For this review, take the finished solid that the model builds, in its own axes (mm). Round coordinates to 2 decimals unless told otherwise and drop trailing zeros. Loops run counter-clockwise (first coordinate to the right, second up) from the corner with the lowest first, then second, coordinate; pieces in that order, holes last.
1) Wall thickness on L1, parallel to X at y = 0.55, z = 19.05 (3 decimals); L2, parallel to Z at x = -28, y = 0.5; L3, parallel to Z at x = 45, y = 0.5: over which ranges is each line inside the solid? List them lowest first.
2) Take a section at A-A (x = -24.5). State the section outline as (y, z) points.
3) Insertion check: pin 1 (8 mm diameter, centred on x = -82.55, z = 39.37, fed in from +Y); pin 2 (3 mm diameter, centred on x = -64.21, z = -39.37, fed in from -Y). Each pin has a flat end and moves straight along its axis. Give the tip position at first contact, or say it passes through.
4) Take a section at B-B (z = 5.5). State the section outline as (x, y) points, then the cut area to 3 significant figures.
5) Take a section at C-C (z = 19.05). Give the number of separate pieces and of enclosed holes in the cut face, then the cut area to 3 significant figures.
```python
from build123d import *

# Parameters (mm, degrees)
SKETCH1_W           = 190.5
SKETCH1_H           = 114.3
BOSS_EXTRUDE1_DEPTH = 1.5875
SKETCH6_W           = 139.7
SKETCH6_H           = 63.5
CUT_EXTRUDE1_DEPTH  = 3.175
FILLET1_R           = 2.54
SKETCH7_R           = 3.175
CUT_EXTRUDE2_DEPTH  = 3.175
SKETCH8_R           = 2.54
CUT_EXTRUDE3_DEPTH  = 2.54
SKETCH9_R           = 2.54
CUT_EXTRUDE4_DEPTH  = 2.54
SKETCH10_W          = 68.58
SKETCH10_H          = 12.7
CUT_EXTRUDE5_DEPTH  = 112.090976934
FILLET2_R           = 2.54


with BuildPart() as part:
    # Sketch1 → Boss-Extrude1 (new body)
    with BuildSketch(Plane(origin=(0, 0, 0), x_dir=(1, 0, 0), z_dir=(0, 1, 0))):
        Rectangle(SKETCH1_W, SKETCH1_H)
    extrude(amount=BOSS_EXTRUDE1_DEPTH)

    # Sketch6 → Cut-Extrude1 (cut)
    with BuildSketch(Plane(origin=(0, 1.5875, 0), x_dir=(1, 0, 0), z_dir=(0, 1, 0))):
        Rectangle(SKETCH6_W, SKETCH6_H)
    extrude(amount=-CUT_EXTRUDE1_DEPTH, mode=Mode.SUBTRACT)

    # Fillet1
    fillet1_edges = [part.edges().sort_by_distance(p)[0] for p in [
        (-69.85, 0.79375, 31.75),
        (-69.85, 0.79375, -31.75),
        (69.85, 0.79375, -31.75),
        (69.85, 0.79375, 31.75),
        (95.25, 0.79375, -57.15),
        (95.25, 0.79375, 57.15),
        (-95.25, 0.79375, 57.15),
        (-95.25, 0.79375, -57.15),
    ]]
    fillet(fillet1_edges, radius=FILLET1_R)

    # Sketch7 → Cut-Extrude2 (cut)
    with BuildSketch(Plane(origin=(0, 1.5875, 0), x_dir=(1, 0, 0), z_dir=(0, 1, 0))):
        with Locations(Location((-82.55, 19.05, 0), (0, 0, 270))):
            Circle(SKETCH7_R)
        with Locations(Location((-82.55, -19.05, 0), (0, 0, 270))):
            Circle(SKETCH7_R)
        with Locations(Location((82.55, -19.05, 0), (0, 0, 270))):
            Circle(SKETCH7_R)
        with Locations(Location((82.55, 19.05, 0), (0, 0, 270))):
            Circle(SKETCH7_R)
    extrude(amount=-CUT_EXTRUDE2_DEPTH, mode=Mode.SUBTRACT)

    # Sketch8 → Cut-Extrude3 (cut)
    with BuildSketch(Plane(origin=(0, 1.5875, 0), x_dir=(1, 0, 0), z_dir=(0, 1, 0))):
        with Locations(Location((82.55, 39.37, 0), (0, 0, 270))):
            Circle(SKETCH8_R)
        with Locations(Location((64.205555556, 39.37, 0), (0, 0, 270))):
            Circle(SKETCH8_R)
        with Locations(Location((45.861111111, 39.37, 0), (0, 0, 270))):
            Circle(SKETCH8_R)
        with Locations(Location((27.516666667, 39.37, 0), (0, 0, 270))):
            Circle(SKETCH8_R)
        with Locations(Location((9.172222222, 39.37, 0), (0, 0, 270))):
            Circle(SKETCH8_R)
        with Locations(Location((-9.172222222, 39.37, 0), (0, 0, 270))):
            Circle(SKETCH8_R)
        with Locations(Location((-27.516666667, 39.37, 0), (0, 0, 270))):
            Circle(SKETCH8_R)
        with Locations(Location((-45.861111111, 39.37, 0), (0, 0, 270))):
            Circle(SKETCH8_R)
        with Locations(Location((-64.205555556, 39.37, 0), (0, 0, 270))):
            Circle(SKETCH8_R)
        with Locations(Location((-82.55, 39.37, 0), (0, 0, 270))):
            Circle(SKETCH8_R)
    extrude(amount=-CUT_EXTRUDE3_DEPTH, mode=Mode.SUBTRACT)

    # Sketch9 → Cut-Extrude4 (cut)
    with BuildSketch(Plane(origin=(0, 1.5875, 0), x_dir=(1, 0, 0), z_dir=(0, 1, 0))):
        with Locations(Location((82.55, -39.37, 0), (0, 0, 270))):
            Circle(SKETCH9_R)
        with Locations(Location((64.205555556, -39.37, 0), (0, 0, 270))):
            Circle(SKETCH9_R)
        with Locations(Location((45.861111111, -39.37, 0), (0, 0, 270))):
            Circle(SKETCH9_R)
        with Locations(Location((27.516666667, -39.37, 0), (0, 0, 270))):
            Circle(SKETCH9_R)
        with Locations(Location((9.172222222, -39.37, 0), (0, 0, 270))):
            Circle(SKETCH9_R)
        with Locations(Location((-9.172222222, -39.37, 0), (0, 0, 270))):
            Circle(SKETCH9_R)
        with Locations(Location((-27.516666667, -39.37, 0), (0, 0, 270))):
            Circle(SKETCH9_R)
        with Locations(Location((-45.861111111, -39.37, 0), (0, 0, 270))):
            Circle(SKETCH9_R)
        with Locations(Location((-64.205555556, -39.37, 0), (0, 0, 270))):
            Circle(SKETCH9_R)
        with Locations(Location((-82.55, -39.37, 0), (0, 0, 270))):
            Circle(SKETCH9_R)
    extrude(amount=-CUT_EXTRUDE4_DEPTH, mode=Mode.SUBTRACT)

    # Sketch10 → Cut-Extrude5 (cut, through all)
    with BuildSketch(Plane(origin=(0, 1.5875, 0), x_dir=(1, 0, 0), z_dir=(0, 1, 0))):
        with Locations((0, -38.1)):
            Rectangle(SKETCH10_W, SKETCH10_H)
        with Locations((0, 38.1)):
            Rectangle(SKETCH10_W, SKETCH10_H)
    extrude(amount=-CUT_EXTRUDE5_DEPTH, mode=Mode.SUBTRACT)

    # Fillet2
    fillet2_edges = [part.edges().sort_by_distance(p)[0] for p in [
        (-34.29, 0.79375, 44.45),
        (-34.29, 0.79375, 31.75),
        (34.29, 0.79375, 31.75),
        (34.29, 0.79375, 44.45),
        (-34.29, 0.79375, -31.75),
        (-34.29, 0.79375, -44.45),
        (34.29, 0.79375, -44.45),
        (34.29, 0.79375, -31.75),
    ]]
    fillet(fillet2_edges, radius=FILLET2_R)


solid = part.part
```
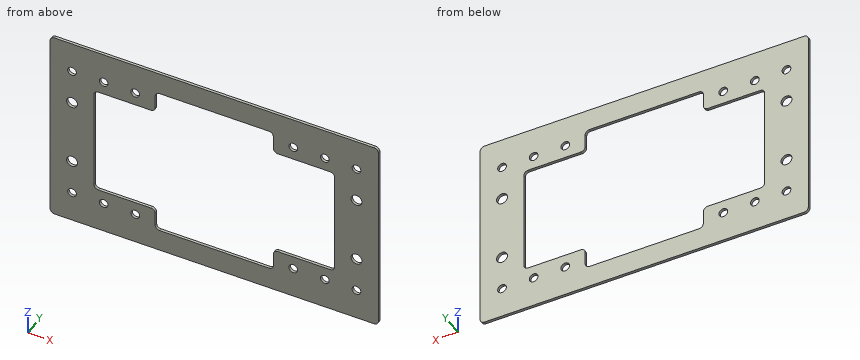
Response:
1. L1: x = -95.25 to -85.725, -79.375 to -69.85, 69.85 to 79.375, 85.725 to 95.25
1. L2: z = -57.15 to -44.45, 44.45 to 57.15
1. L3: z = -57.15 to -41.76, -36.98 to -31.75, 31.75 to 36.98, 41.76 to 57.15
2. outline: (0, -57.15) - (1.59, -57.15) - (1.59, -44.45) - (0, -44.45) - close; (0, 44.45) - (1.59, 44.45) - (1.59, 57.15) - (0, 57.15) - close
3. pin 1: stops at y = 1.59
3. pin 2: passes through
4. outline: (-95.25, 0) - (-69.85, 0) - (-69.85, 1.59) - (-95.25, 1.59) - close; (69.85, 0) - (95.25, 0) - (95.25, 1.59) - (69.85, 1.59) - close
4. area: 80.6 mm2
5. separate pieces: 4
5. enclosed holes: 0
5. area: 60.5 mm2
